Input: part model. Units: mm. Frame: model coordinates. Face numbers are marked on the shaded views. A direction names the side the tool comes from. Coordinates: 2 decimals unless noted, no trailing zeros. Order: outer loops, then holes, each group sorted by start corner. A loop starts at its lowest first (then second) coordinate and runs counter-clockwise, first axis right, second up. Notation, with made-up numbers: (45.5, -16.75) -> (64.5, -16.75) arc R9 ccw to (64.5, -5.75) -> close; hole circle Ø7 at (48.5, 79.25). An arc over 180 degrees is marked (long way). One line per item, written item: value. Start each with the question number.
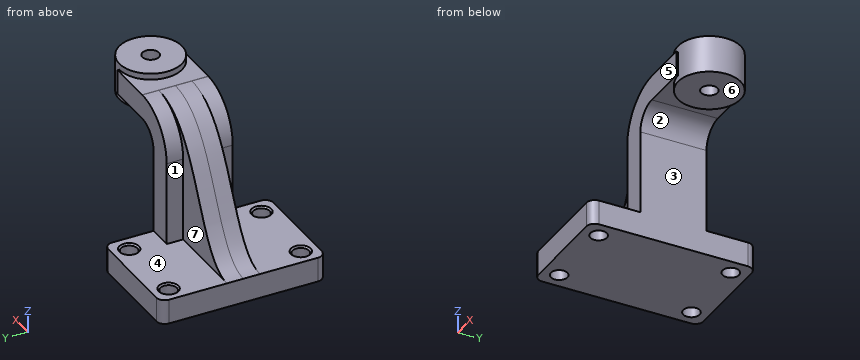
from build123d import *

# Parameters (mm, degrees)
F1_DEPTH       = 63.5
F0_W           = 26.6882655859
F0_H           = 19.05
F2_DEPTH       = 25.4
F3_DEPTH       = 12.7
F5_R           = 6.35
F7_D           = 12.7
F9_D           = 12.7
F9_CSINK_D     = 15.24
F9_CSINK_ANGLE = 90


with BuildPart() as f1:
    # F0 (on Front) → F1 (new body, symmetric)
    with BuildSketch(Plane.XZ):
        Polygon((-41.275, 9.525), (-41.275, -9.525), (41.275, -9.525), (41.275, 9.525), (22.225, 9.525), align=None)
    extrude(amount=F1_DEPTH, both=True)

    # F0 (on Front) → F2 (join, symmetric)
    with BuildSketch(Plane.XZ):
        with BuildLine():
            Line((22.225, 9.525), (41.275, 9.525))
            Line((41.275, 9.525), (41.275, 73.9775))
            ThreePointArc((41.275, 73.9775), (46.1106670426, 85.6518329574), (57.785, 90.4875))
            Line((57.785, 90.4875), (66.675, 90.4875))
            Line((66.675, 90.4875), (66.675, 109.5375))
            Line((66.675, 109.5375), (57.785, 109.5375))
            add(Edge.make_bspline(
                [(57.3658867379, 109.5350300615), (57.5052527002, 109.5364377458), (57.6449566509, 109.5372620063), (57.785, 109.5375)],
                knots=[140.4259734343, 140.4259734343, 140.4259734343, 140.4259734343, 140.7671259785, 140.7671259785, 140.7671259785, 140.7671259785], degree=3))
            ThreePointArc((57.3658867379, 109.5350300615), (32.4925380044, 98.9735990196), (22.225, 73.9775))
            Line((22.225, 73.9775), (22.225, 9.525))
        make_face()
        with Locations((80.019132793, 100.0125)):
            Rectangle(F0_W, F0_H)
    extrude(amount=F2_DEPTH, both=True)

    # F0 (on Front) → F3 (join, symmetric)
    with BuildSketch(Plane.XZ):
        with BuildLine():
            add(Edge.make_bspline(
                [(-41.275, 9.525), (-0.1000309637, 9.525), (-0.0002424275, 108.9555959023), (57.3658867379, 109.5350300615)],
                knots=[0, 0, 0, 0, 140.4259734343, 140.4259734343, 140.4259734343, 140.4259734343], degree=3))
            Line((-41.275, 9.525), (22.225, 9.525))
            Line((22.225, 9.525), (22.225, 73.9775))
            ThreePointArc((22.225, 73.9775), (32.4925380044, 98.9735990196), (57.3658867379, 109.5350300615))
        make_face()
    extrude(amount=F3_DEPTH, both=True)

    # F0 (on Front) → F4 (revolve)
    with BuildSketch(Plane.XZ):
        Polygon((93.3632655859, 114.3), (93.3632655859, 109.5375), (93.3632655859, 90.4875), (93.3632655859, 85.725), (117.475, 85.725), (117.475, 114.3), align=None)
    revolve(axis=Axis((93.3632655859, 0, 100.0125), (0, 0, 1)))

    # F5
    f5_edges = [f1.edges().sort_by_distance(p)[0] for p in [
        (-41.275, -63.5, 0),
        (41.275, -63.5, 0),
        (-41.275, 63.5, 0),
        (41.275, 63.5, 0),
    ]]
    fillet(f5_edges, radius=F5_R)

    # F7 (through all)
    with Locations(Plane.XY.offset(114.3)):
        with Locations((93.3632655859, 0)):
            Hole(F7_D / 2)

    # F9 (through all)
    with Locations(Plane.XY.offset(9.525)):
        with Locations((-28.575, -50.8), (28.575, -50.8), (28.575, 50.8), (-28.575, 50.8)):
            CounterSinkHole(F9_D / 2, F9_CSINK_D / 2, counter_sink_angle=F9_CSINK_ANGLE)


solid = f1.part
1) Section query B-B, the plane x = 28. State how many separate pieces and enclosed holes the cut face has, plus the area to 3 significant figures.
2) Pin query (flat end, axial travel): pin 1 Ø6 at (x, y) = (83, -4) entering from -Z (3 decimals); pin 2 Ø3 at (x, z) = (27, 72.5) entering from -Y; pin 3 Ø1.5 at (y, z) = (15, 57) entering from -X (3 decimals); pin 4 Ø11.5 at (x, y) = (28.575, 50.8) entering from -Z. Return the tip coordinate at first contact, or that it passes through.
3) Ray query, line 1 along X through (y, z) = (50.8, -0.75) (3 decimals); line 2 along Z through (x, y) = (10.5, 56.5) (3 decimals); line 3 along X through (y, z) = (55, 3.5) (3 decimals). Return the intervals inside material, ascending. Write a range as from..to.
4) Mould query, pull axis X, two halves, no side actions, for the marked faces 1, 2, 3 and 4. Classes: +X half, -X half, draft (parallel to the pull), parting line (faces both ways), or undercut.
5) Section query A-A, the plane y = 50.8. Return the cut outline in (x, z) (3 decimals).
6) Access query for the marked faces 5, 6 and 7. Directions: +Z, -Z, +X, -X, +Y, -Y. A direction counts if a zero-diameter tool reaches every point of the face in a straight line with its end or side. Return the directions, or none.
Entries:
1. separate pieces: 3
1. enclosed holes: 0
1. area: 6,310 mm2
2. pin 1: stops at z = 85.725
2. pin 2: stops at y = -25.4
2. pin 3: stops at x = 22.225
2. pin 4: passes through
3. line 1: x = -41.275..-34.925, -22.225..22.225, 34.925..41.275
3. line 2: z = -9.525..9.525
3. line 3: x = -41.275..-33.338, -23.812..23.812, 33.338..41.275
4. face 1: -X half
4. face 2: undercut
4. face 3: +X half
4. face 4: draft
5. outline: (-41.275, -9.525) -> (-34.925, -9.525) -> (-34.925, 8.255) -> (-36.195, 9.525) -> (-41.275, 9.525) -> close; (-22.225, -9.525) -> (22.225, -9.525) -> (22.225, 8.255) -> (20.955, 9.525) -> (-20.955, 9.525) -> (-22.225, 8.255) -> close; (34.925, -9.525) -> (41.275, -9.525) -> (41.275, 9.525) -> (36.195, 9.525) -> (34.925, 8.255) -> close
6. face 5: +Z, +X, -X, -Y
6. face 6: -Z, +X, +Y, -Y
6. face 7: +Z, -X, +Y
